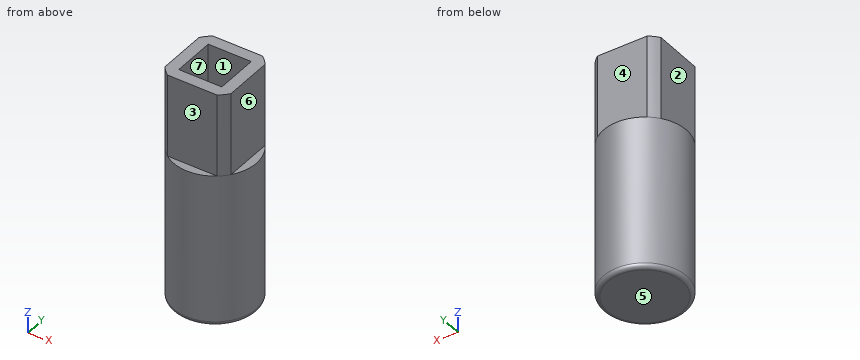
from build123d import *

# Parameters (mm, degrees)
SKETCH1_R           = 5
BOSS_EXTRUDE1_DEPTH = 18.5
BOSS_EXTRUDE2_DEPTH = 10
SKETCH4_W           = 5.2
SKETCH4_H           = 5.2
CUT_EXTRUDE2_DEPTH  = 10
FILLET1_R           = 0.5


with BuildPart() as part:
    # Sketch1 → Boss-Extrude1 (new body)
    with BuildSketch(Plane.XY):
        Circle(SKETCH1_R)
    extrude(amount=BOSS_EXTRUDE1_DEPTH)

    # Sketch3 → Boss-Extrude2 (add)
    with BuildSketch(Plane.XY.offset(18.5)):
        with BuildLine():
            ThreePointArc((-4, -3), (-3.535533906, -3.535533906), (-3, -4))
            Line((-3, -4), (3, -4))
            ThreePointArc((3, -4), (3.535533906, -3.535533906), (4, -3))
            Line((4, -3), (4, 3))
            ThreePointArc((4, 3), (3.535533906, 3.535533906), (3, 4))
            Line((3, 4), (-3, 4))
            ThreePointArc((-3, 4), (-3.535533906, 3.535533906), (-4, 3))
            Line((-4, 3), (-4, -3))
        make_face()
    extrude(amount=BOSS_EXTRUDE2_DEPTH)

    # Sketch4 → Cut-Extrude2 (cut)
    with BuildSketch(Plane.XY.offset(28.5)):
        Rectangle(SKETCH4_W, SKETCH4_H)
    extrude(amount=-CUT_EXTRUDE2_DEPTH, mode=Mode.SUBTRACT)

    # Fillet1
    fillet1_edges = [part.edges().sort_by_distance(p)[0] for p in [
        (-5, 0, 0),
    ]]
    fillet(fillet1_edges, radius=FILLET1_R)


solid = part.part
Can you work these out from the model? Positions are in its coordinate system, mm. Face numbers are marked on the shaded views. A direction names the side the tool comes from. Round coordinates to 2 decimals unless told otherwise and drop trailing zeros. Loops run counter-clockwise (first coordinate to the right, second up) from the corner with the lowest first, then second, coordinate; pieces in that order, holes last. Notation, with made-up numbers: (2, 46.25) - (8, 46.25) arc R20 cw to (8, 74.25) - close; hole circle Ø11 at (73.5, 11.25). An arc over 180 degrees is marked (long way). Use CSV: the item, a comma, the result in double quotes. Start each with the question number.
1) If we section it at A-A on y = 0: Write out the boundary of the cut face in (x, z), plus the area to 3 significant figures.
2) If we section it at C-C on z = 14: Write out the boundary of the cut face in (x, y), plus the area to 3 significant figures.
3) Please list where these lines run through material, in increasing order: probe 1 along Y at (x, z) = (-2, 25); probe 2 along Z at (x, y) = (0, -1.5). Write a range as [from, to].
4) We'd pull the mould along Y, two halves only. Please class the marked faces 1, 2, 3 and 4: released by +Y, released by -Y, zero draft, split by the parting line, or undercut.
5) For pin 1 Ø5 at (x, z) = (0, 25) entering from +Y; pin 2 Ø1.8 at (y, z) = (1, 25) entering from -X; pin 3 Ø0.8 at (x, y) = (4.5, -0.5) entering from +Z, each with a flat end and sliding along its axis, tell me the tip position at first contact or that it passes through.
6) For the marked faces 5, 6 and 7, which set-ups out of +Z, -Z, +X, -X, +Y, -Y let a thin tool reach every point of the face, with its end or its side?
Geometry results:
1,outline,"(-5, 0.5) arc R0.5 ccw to (-4.5, 0) - (4.5, 0) arc R0.5 ccw to (5, 0.5) - (5, 18.5) - (4, 18.5) - (4, 28.5) - (2.6, 28.5) - (2.6, 18.5) - (-2.6, 18.5) - (-2.6, 28.5) - (-4, 28.5) - (-4, 18.5) - (-5, 18.5) - close"
1,area,"213 mm2"
2,outline,"circle Ø10 at (0, 0)"
2,area,"78.5 mm2"
3,probe 1,"y = [-4, -2.6], [2.6, 4]"
3,probe 2,"z = [0, 18.5]"
4,face 1,"undercut"
4,face 2,"zero draft"
4,face 3,"released by -Y"
4,face 4,"released by +Y"
5,pin 1,"stops at y = 4"
5,pin 2,"stops at x = -4"
5,pin 3,"stops at z = 18.5"
6,face 5,"-Z, +X, -X, +Y, -Y"
6,face 6,"+Z, +X, +Y, -Y"
6,face 7,"+Z"
